Check sheet for the modelled part. Datum: model origin and axes. Units: mm. Face numbers are marked on the shaded views. A direction names the side the tool comes from. Round coordinates to 2 decimals unless told otherwise and drop trailing zeros. Write each loop counter-clockwise with the first axis right and the second up, starting at its lowest first coordinate (ties: lowest second). Pieces come first, ordered by that corner, then holes.
Item 1: Cross-section at B-B on y = 0. Enter the section's corners in (x, z), plus the area to 3 significant figures.
Item 2: Tool access check on the marked faces 1 and 2. Record the directions out of +Z, -Z, +X, -X, +Y, -Y that give a thin tool (end or side, any length) a straight path to the whole face; none if there is none.
Item 3: Go/stop test with a flat-tipped pin: pin 1 Ø6 at (y, z) = (-14, -4) entering from -X. Record where the tip stops, or that it passes through.
Item 4: Cross-section at A-A on z = -6.5. Enter the section's corners in (x, y) (3 decimals), plus the area to 3 significant figures.
Item 5: Material ranges on line 1 (Y direction, x = 20, z = -11.5) (3 decimals); line 2 (Z direction, x = 14, y = -12), recorded low to high.
from build123d import *

# Parameters (mm, degrees)
SKETCH1_W                      = 50.8
SKETCH1_H                      = 41.91
BASE_FLANGE1_DEPTH             = 0.762
EDGE_FLANGE1_STRIP_W           = 3.81
EDGE_FLANGE1_STRIP_H           = 0.762
EDGE_FLANGE1_STRIP_CUT_DEPTH   = 50.8
EDGE_FLANGE1_STRIP_2_W         = 3.81
EDGE_FLANGE1_STRIP_2_H         = 0.762
EDGE_FLANGE1_STRIP_CUT_2_DEPTH = 50.8
EDGE_FLANGE1_DEPTH             = 50.8
EDGE_FLANGE1_BEND_DEPTH        = 50.8
SKETCH14_R                     = 18.415
CUT_EXTRUDE1_DEPTH             = 2.54
SKETCH16_R                     = 0.4445
CUT_EXTRUDE4_DEPTH             = 53.848
SKETCH17_R                     = 2.1082
CUT_EXTRUDE5_DEPTH             = 36.025531673
CUT_EXTRUDE6_DEPTH             = 36.025531673


# Sheet-metal steps are written as plain solids
with BuildPart() as part:
    # Sketch1 → Base-Flange1 (new body)
    with BuildSketch(Plane.XY):
        Rectangle(SKETCH1_W, SKETCH1_H)
    extrude(amount=-BASE_FLANGE1_DEPTH)

    # Edge-Flange1 strip (across the edge) → Edge-Flange1 strip cut (cut)
    with BuildSketch(Plane(origin=(-25.4, 20.955, -0.762), x_dir=(0, -1, 0), z_dir=(1, 0, 0))):
        with Locations((-0.762, -0.381)):
            Rectangle(EDGE_FLANGE1_STRIP_W, EDGE_FLANGE1_STRIP_H)
    extrude(amount=EDGE_FLANGE1_STRIP_CUT_DEPTH, mode=Mode.SUBTRACT)

    # Edge-Flange1 strip 2 (across the edge) → Edge-Flange1 strip cut 2 (cut)
    with BuildSketch(Plane(origin=(25.4, -20.955, -0.762), x_dir=(0, 1, 0), z_dir=(-1, 0, 0))):
        with Locations((-0.762, -0.381)):
            Rectangle(EDGE_FLANGE1_STRIP_2_W, EDGE_FLANGE1_STRIP_2_H)
    extrude(amount=EDGE_FLANGE1_STRIP_CUT_2_DEPTH, mode=Mode.SUBTRACT)

    # Edge-Flange1 section (across the edge) → Edge-Flange1 (add)
    with BuildSketch(Plane(origin=(-25.4, 20.955, -0.762), x_dir=(0, -1, 0), z_dir=(1, 0, 0))):
        with BuildLine():
            Line((0, 0.381), (0, 11.938))
            Line((0, 11.938), (0.762, 11.938))
            Line((0.762, 11.938), (0.762, 0.381))
            ThreePointArc((0.762, 0.381), (0.873592316, 0.111592316), (1.143, 0))
            Line((1.143, 0), (1.143, -0.762))
            ThreePointArc((1.143, -0.762), (0.334776949, -0.427223051), (0, 0.381))
        make_face()
    extrude(amount=EDGE_FLANGE1_DEPTH)

    # Edge-Flange1 section 2 (across the edge) → Edge-Flange1 bend (add)
    with BuildSketch(Plane(origin=(25.4, -20.955, -0.762), x_dir=(0, 1, 0), z_dir=(-1, 0, 0))):
        with BuildLine():
            Line((0, 0.381), (0, 11.938))
            Line((0, 11.938), (0.762, 11.938))
            Line((0.762, 11.938), (0.762, 0.381))
            ThreePointArc((0.762, 0.381), (0.873592316, 0.111592316), (1.143, 0))
            Line((1.143, 0), (1.143, -0.762))
            ThreePointArc((1.143, -0.762), (0.334776949, -0.427223051), (0, 0.381))
        make_face()
    extrude(amount=EDGE_FLANGE1_BEND_DEPTH)

    # Sketch14 → Cut-Extrude1 (cut)
    with BuildSketch(Plane.XY.offset(0.889)):
        with Locations(Location((-3.954996568, 0, 0), (0, 0, 180))):
            Circle(SKETCH14_R)
    extrude(amount=-CUT_EXTRUDE1_DEPTH, mode=Mode.SUBTRACT)

    # Sketch16 → Cut-Extrude4 (cut)
    with BuildSketch(Plane(origin=(0, 20.955, 0), x_dir=(1, 0, 0), z_dir=(0, 1, 0))):
        with Locations(Location((22.225, 9.525, 0), (0, 0, 270))):
            Circle(SKETCH16_R)
        with Locations(Location((-22.225, 9.525, 0), (0, 0, 270))):
            Circle(SKETCH16_R)
    extrude(amount=-CUT_EXTRUDE4_DEPTH, mode=Mode.SUBTRACT)

    # Sketch17 → Cut-Extrude5 (cut, through all)
    with BuildSketch(Plane(origin=(0, 0, -0.762), x_dir=(-1, 0, 0), z_dir=(0, 0, -1))):
        with Locations((-22.225, 15.875)):
            Circle(SKETCH17_R)
        with Locations((-22.225, -15.875)):
            Circle(SKETCH17_R)
        with Locations((22.225, -15.875)):
            Circle(SKETCH17_R)
        with Locations((22.225, 15.875)):
            Circle(SKETCH17_R)
    extrude(amount=-CUT_EXTRUDE5_DEPTH, mode=Mode.SUBTRACT)

    # Sketch18 → Cut-Extrude6 (cut, through all)
    with BuildSketch(Plane(origin=(0, 0, -0.762), x_dir=(-1, 0, 0), z_dir=(0, 0, -1))):
        with BuildLine():
            Line((-10.968730797, 10.788632283), (-22.86, 10.788632283))
            Line((-22.86, 10.788632283), (-22.86, -10.788632283))
            Line((-22.86, -10.788632283), (-10.968730797, -10.788632283))
            ThreePointArc((-10.968730797, -10.788632283), (-14.460003432, 0), (-10.968730797, 10.788632283))
        make_face()
    extrude(amount=-CUT_EXTRUDE6_DEPTH, mode=Mode.SUBTRACT)


solid = part.part
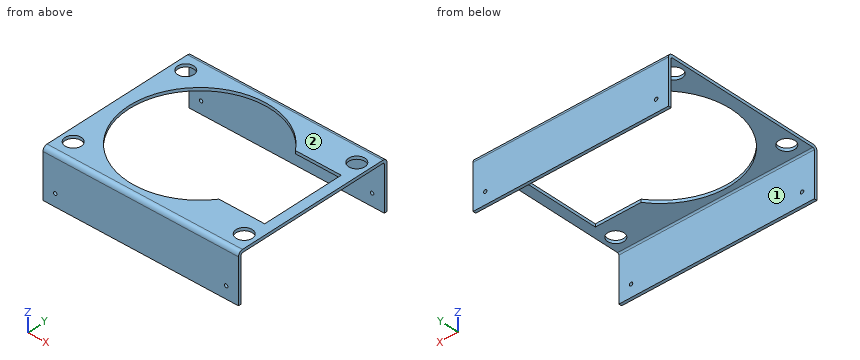
Response values:
1. outline: (-25.4, -0.76) - (-22.37, -0.76) - (-22.37, 0) - (-25.4, 0) - close; (22.86, -0.76) - (25.4, -0.76) - (25.4, 0) - (22.86, 0) - close
1. area: 4.24 mm2
2. face 1: -Z, +X, -X
2. face 2: +Z, +X, -X, +Y, -Y
3. pin 1: passes through
4. outline: (-25.4, -20.955) - (25.4, -20.955) - (25.4, -20.193) - (-25.4, -20.193) - close; (-25.4, 20.193) - (25.4, 20.193) - (25.4, 20.955) - (-25.4, 20.955) - close
4. area: 77.4 mm2
5. line 1: y = -20.955 to -20.193, 20.193 to 20.955
5. line 2: z = -0.76 to 0
